```python
from build123d import *

# Parameters (mm, degrees)
SKETCH1_R               = 5.1
SKETCH1_R_2             = 2.3
BOSS_EXTRUDE1_DEPTH     = 25
SKETCH4_W               = 50
SKETCH4_H               = 12.5
BOSS_EXTRUDE3_DEPTH     = 4
CUT_EXTRUDE3_DEPTH      = 87.900747983
CUT_EXTRUDE3_DEPTH_BACK = 87.900747983
SKETCH5_R               = 1.8
CUT_EXTRUDE4_DEPTH      = 87.900747983
CUT_EXTRUDE4_DEPTH_BACK = 10


with BuildPart() as part:
    # Sketch1 → Boss-Extrude1 (new body)
    with BuildSketch(Plane(origin=(0, 0, 0), x_dir=(1, 0, 0), z_dir=(0, 1, 0))):
        with BuildLine():
            Line((30, 12.5), (30, -12.5))
            Line((30, -12.5), (30, -25))
            Line((30, -25), (26, -25))
            Line((26, -25), (-3.605153395, -14.630751305))
            Line((-3.605153395, -14.630751305), (-35.757725948, -9.893181241))
            ThreePointArc((-35.757725948, -9.893181241), (-44.3, 0), (-35.757725948, 9.893181241))
            Line((-35.757725948, 9.893181241), (-3.605153395, 14.630751305))
            Line((-3.605153395, 14.630751305), (26, 25))
            Line((26, 25), (30, 25))
            Line((30, 25), (30, 12.5))
        make_face()
        with Locations(Location((0, 0, 0), (0, 0, 270))):
            Circle(SKETCH1_R, mode=Mode.SUBTRACT)
        with Locations(Location((-34.3, 0, 0), (0, 0, 270))):
            Circle(SKETCH1_R_2, mode=Mode.SUBTRACT)
    extrude(amount=BOSS_EXTRUDE1_DEPTH)

    # Sketch4 → Boss-Extrude3 (add)
    with BuildSketch(Plane(origin=(30, 0, 0), x_dir=(0, 0, -1), z_dir=(1, 0, 0))):
        with Locations((0, 31.25)):
            Rectangle(SKETCH4_W, SKETCH4_H)
        with Locations((0, -6.25)):
            Rectangle(SKETCH4_W, SKETCH4_H)
    extrude(amount=-BOSS_EXTRUDE3_DEPTH)

    # Sketch5 → Cut-Extrude3 (cut, two sides: drawn at the far end of the back side and taken through both)
    with BuildSketch(Plane(origin=(30, 0, 0), x_dir=(0, 0, -1), z_dir=(1, 0, 0)).offset(-CUT_EXTRUDE3_DEPTH_BACK)):
        with Locations(Location((-17.5, 31.5, 0), (0, 0, 180))):
            Circle(SKETCH5_R)
        with Locations(Location((17.5, 31.5, 0), (0, 0, 180))):
            Circle(SKETCH5_R)
        with Locations(Location((17.5, -6.5, 0), (0, 0, 180))):
            Circle(SKETCH5_R)
        with Locations(Location((-17.5, -6.5, 0), (0, 0, 180))):
            Circle(SKETCH5_R)
    extrude(amount=CUT_EXTRUDE3_DEPTH + CUT_EXTRUDE3_DEPTH_BACK, mode=Mode.SUBTRACT)

    # Sketch3 → Cut-Extrude4 (cut, two sides: drawn at the far end of the back side and taken through both)
    with BuildSketch(Plane(origin=(30, 0, 0), x_dir=(0, 0, -1), z_dir=(1, 0, 0)).offset(-CUT_EXTRUDE4_DEPTH_BACK)):
        Polygon((-4.965212315, 21.1), (-9.93042463, 12.5), (-4.965212315, 3.9), (4.965212315, 3.9), (9.93042463, 12.5), (4.965212315, 21.1), align=None)
    extrude(amount=CUT_EXTRUDE4_DEPTH + CUT_EXTRUDE4_DEPTH_BACK, mode=Mode.SUBTRACT)


solid = part.part
```
Part model, mm, in its own coordinate system. A direction names the side the tool comes from. Coordinates: 2 decimals unless noted, no trailing zeros. Loops run counter-clockwise (first coordinate to the right, second up) from the corner with the lowest first, then second, coordinate; pieces in that order, holes last. Notation, with made-up numbers: (-15, 64.25) - (44, 64.25) arc R28 ccw to (44, 102.25) - close; hole circle Ø7 at (9.25, -8.5). An arc over 180 degrees is marked (long way). Write item = value, one per line. Start each with the question number.
Item 1: Flat gauge pins, fed straight in: pin 1 Ø2 at (y, z) = (-6.5, -17.5) entering from +X; pin 2 Ø6 at (y, z) = (31.5, 17.5) entering from -X; pin 3 Ø5 at (y, z) = (16.5, -1.5) entering from +X; pin 4 Ø4 at (y, z) = (4.5, 4.5) entering from -X. Where does each tip first touch, or does it go through?
Item 2: Cut at D-D, the plane y = 15. Give the cut face in (x, z).
Item 3: Cut at A-A, the plane y = 31.5. Give the cut face in (x, z), and give its area (3 significant figures).
Item 4: Cut at C-C, the plane x = -34.3. Give the cut face in (y, z), and give its area (3 significant figures).
Item 5: Cut at B-B, the plane z = 0. Give the cut face in (x, y), and give its area (3 significant figures).
Item 6: 3-axis set-ups, long thin cutter, end or side, ignore diameter. For faces 1 (the flat face through (24.93, 8.26, 7.483)), 2 (the flat face through (26, -6, 0)), 3 (the flat face through (-1, 25, -6)): which of +Z, -Z, +X, -X, +Y, -Y reach the whole face in a straight line?
Item 7: Mould opens along Y. For faces 4 (the flat face through (30, 24, 0)), 5 (the flat face through (28, -12.5, 0)), 6 (the cylindrical face through (27.972, 29.715, -17.734)), 7 (the flat face through (28, 37.5, 0)) say: released by +Y, released by -Y, zero draft, split by the parting line, or undercut.
Item 8: Wall check: L1, parallel to X at y = 19, z = 0; L2, parallel to Y at x = 28.2, z = 17.5; L3, parallel to X at y = 14, z = -1.5. Give the ranges that are in metal, low to high. Write a range as from..to.
The answers:
q1.pin_1 = through
q1.pin_2 = 26
q1.pin_3 = 20
q1.pin_4 = -43.98
q2.outline = (-35.76, -9.89) - (-3.61, -14.63) - (26, -25) - (30, -25) - (30, -8.49) - (20, -8.49) - (20, 8.49) - (30, 8.49) - (30, 25) - (26, 25) - (-3.61, 14.63) - (-35.76, 9.89) arc R10 ccw to start; hole circle Ø4.6 at (-34.3, 0); hole circle Ø10.2 at (0, 0)
q3.outline = (26, -25) - (30, -25) - (30, -19.3) - (26, -19.3) - close; (26, -15.7) - (30, -15.7) - (30, 15.7) - (26, 15.7) - close; (26, 19.3) - (30, 19.3) - (30, 25) - (26, 25) - close
q3.area = 171 mm2
q4.outline = (0, -10.11) - (25, -10.11) - (25, -2.3) - (0, -2.3) - close; (0, 2.3) - (25, 2.3) - (25, 10.11) - (0, 10.11) - close
q4.area = 390 mm2
q5.outline = (-44.3, 0) - (-36.6, 0) - (-36.6, 25) - (-44.3, 25) - close; (-32, 0) - (-5.1, 0) - (-5.1, 25) - (-32, 25) - close; (5.1, 0) - (26, 0) - (26, -12.5) - (30, -12.5) - (30, 3.9) - (20, 3.9) - (20, 21.1) - (30, 21.1) - (30, 37.5) - (26, 37.5) - (26, 25) - (5.1, 25) - close
q5.area = 1,420 mm2
q6.face_1 = +X
q6.face_2 = +Z, -Z, -X, -Y
q6.face_3 = +Z, -Z, -X, +Y
q7.face_4 = zero draft
q7.face_5 = released by -Y
q7.face_6 = undercut
q7.face_7 = released by +Y
q8.L1 = -44.3..-36.6, -32..-5.1, 5.1..20
q8.L2 = -12.5..-8.3, -4.7..29.7, 33.3..37.5
q8.L3 = -44.19..-36.04, -32.56..-4.87, 4.87..20
